The listing builds one solid part. Answer for the finished solid, in the listing's coordinates (mm). Round coordinates to 2 decimals unless told otherwise and drop trailing zeros. Write each loop counter-clockwise with the first axis right and the second up, starting at its lowest first coordinate (ties: lowest second). Pieces come first, ordered by that corner, then holes. Notation, with made-up numbers: (26, -38) - (49, -38) arc R27 ccw to (49, -14) - close; hole circle Ø6 at (17, 18). An arc over 180 degrees is marked (long way). Answer in a Markdown table with one row per item.
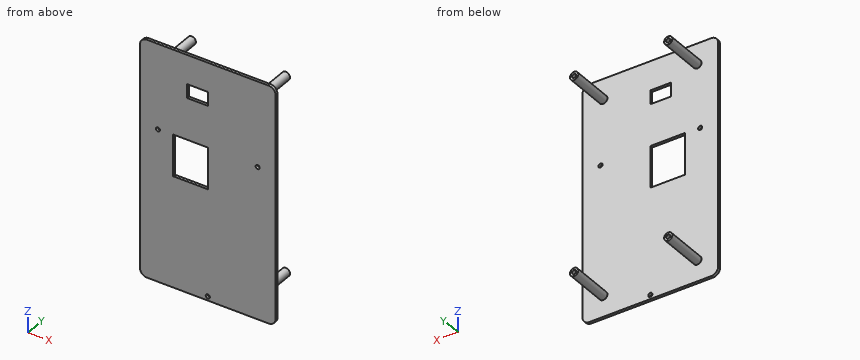
from build123d import *

# Parameters (mm, degrees)
CROQUIS1_W              = 98
CROQUIS1_H              = 171
CROQUIS1_W_2            = 15
CROQUIS1_H_2            = 10
SALIENTE_EXTRUIR1_DEPTH = 2
REDONDEO1_R             = 5
CROQUIS2_R              = 1.5
CORTAR_EXTRUIR2_DEPTH   = 10
CROQUIS5_R              = 3
SALIENTE_EXTRUIR2_DEPTH = 31
CROQUIS6_R              = 1.5
CORTAR_EXTRUIR3_DEPTH   = 15


with BuildPart() as part:
    # Croquis1 → Saliente-Extruir1 (new body)
    with BuildSketch(Plane(origin=(0, 0, 0), x_dir=(1, 0, 0), z_dir=(0, 1, 0))):
        Rectangle(CROQUIS1_W, CROQUIS1_H)
        with Locations((-7.5, -59.5)):
            Rectangle(CROQUIS1_W_2, CROQUIS1_H_2, mode=Mode.SUBTRACT)
        Polygon((-25, 5.5), (0, 5.5), (0, 0), (0, -24.5), (-25, -24.5), align=None, mode=Mode.SUBTRACT)
    extrude(amount=SALIENTE_EXTRUIR1_DEPTH)

    # Redondeo1
    redondeo1_edges = [part.edges().sort_by_distance(p)[0] for p in [
        (49, 1, 85.5),
        (-49, 1, 85.5),
        (-49, 1, -85.5),
        (49, 1, -85.5),
    ]]
    fillet(redondeo1_edges, radius=REDONDEO1_R)

    # Croquis2 → Cortar-Extruir2 (cut)
    with BuildSketch(Plane(origin=(0, 2, 0), x_dir=(1, 0, 0), z_dir=(0, 1, 0))):
        with Locations(Location((-36, -24, 0), (0, 0, 270))):
            Circle(CROQUIS2_R)
        with Locations(Location((36, -24, 0), (0, 0, 270))):
            Circle(CROQUIS2_R)
        with Locations(Location((0, 82.5, 0), (0, 0, 270))):
            Circle(CROQUIS2_R)
    extrude(amount=-CORTAR_EXTRUIR2_DEPTH, mode=Mode.SUBTRACT)

    # Croquis5 → Saliente-Extruir2 (add)
    with BuildSketch(Plane(origin=(0, 2, 0), x_dir=(1, 0, 0), z_dir=(0, 1, 0))):
        with Locations(Location((-34, 70.5, 0), (0, 0, 270))):
            Circle(CROQUIS5_R)
        with Locations(Location((34, 70.5, 0), (0, 0, 90))):
            Circle(CROQUIS5_R)
        with Locations(Location((34, -70.5, 0), (0, 0, 270))):
            Circle(CROQUIS5_R)
        with Locations(Location((-34, -70.5, 0), (0, 0, 90))):
            Circle(CROQUIS5_R)
    extrude(amount=SALIENTE_EXTRUIR2_DEPTH)

    # Croquis6 → Cortar-Extruir3 (cut)
    with BuildSketch(Plane(origin=(0, 33, 0), x_dir=(1, 0, 0), z_dir=(0, 1, 0))):
        with Locations(Location((-34, 70.5, 0), (0, 0, 270))):
            Circle(CROQUIS6_R)
        with Locations(Location((34, 70.5, 0), (0, 0, 270))):
            Circle(CROQUIS6_R)
        with Locations(Location((34, -70.5, 0), (0, 0, 270))):
            Circle(CROQUIS6_R)
        with Locations(Location((-34, -70.5, 0), (0, 0, 270))):
            Circle(CROQUIS6_R)
    extrude(amount=-CORTAR_EXTRUIR3_DEPTH, mode=Mode.SUBTRACT)


solid = part.part
(1) Section C-C (z = 15.5) is taken. Give the vertices of the cut face in (x, y).
Checked values:
| item | result |
|---|---|
| outline | (-49, 0) - (-25, 0) - (-25, 2) - (-49, 2) - close; (0, 0) - (49, 0) - (49, 2) - (0, 2) - close |
(2) Section A-A (x = -17.5) is taken. Give the vertices of the cut face in (y, z).
Checked values:
| item | result |
|---|---|
| outline | (0, -85.5) - (2, -85.5) - (2, -5.5) - (0, -5.5) - close; (0, 24.5) - (2, 24.5) - (2, 85.5) - (0, 85.5) - close |
(3) Flat-ended cylindrical pins translate along their axes: pin 1 (2.5 mm diameter, centred on x = 33.5, z = -71, fed in from +Y); pin 2 (1 mm diameter, centred on x = -32, y = 10.5, fed in from +Z); pin 3 (3 mm diameter, centred on x = -30.5, y = 21.5, fed in from -Z); pin 4 (1.8 mm diameter, centred on x = -36, z = 24, fed in from +Y). Find the tip coordinate at first contact, or state that the pin passes through.
Checked values:
| item | result |
|---|---|
| pin 1 | stops at y = 33 |
| pin 2 | stops at z = 73.1 |
| pin 3 | stops at z = -72.74 |
| pin 4 | passes through |
(4) Section B-B (y = 21.5) is taken. Give the vertices of the cut face in (x, z), and give its area (3 significant figures).
Checked values:
| item | result |
|---|---|
| outline | circle Ø6 at (-34, -70.5); circle Ø6 at (-34, 70.5); circle Ø6 at (34, -70.5); circle Ø6 at (34, 70.5); hole circle Ø3 at (-34, -70.5); hole circle Ø3 at (-34, 70.5); hole circle Ø3 at (34, -70.5); hole circle Ø3 at (34, 70.5) |
| area | 84.8 mm2 |
(5) Section D-D (y = 5.5) is taken. Give the vertices of the cut face in (x, z), and give its area (3 significant figures).
Checked values:
| item | result |
|---|---|
| outline | circle Ø6 at (-34, -70.5); circle Ø6 at (-34, 70.5); circle Ø6 at (34, -70.5); circle Ø6 at (34, 70.5) |
| area | 113 mm2 |
(6) Find the intervals of material crossed by line 1 (X direction, y = 23.75, z = 70.5); line 2 (X direction, y = 29, z = -70); line 3 (Y direction, x = -28, z = -21.5), in increasing order.
Checked values:
| item | result |
|---|---|
| line 1 | x = -37 to -35.5, -32.5 to -31, 31 to 32.5, 35.5 to 37 |
| line 2 | x = -36.96 to -35.41, -32.59 to -31.04, 31.04 to 32.59, 35.41 to 36.96 |
| line 3 | y = 0 to 2 |
